```python
from build123d import *

# Parameters (mm, degrees)
SKETCH_1_W           = 30
SKETCH_1_H           = 30
EXTRUDE_1_DEPTH      = 30
SKETCH_34_W          = 20
SKETCH_34_H          = 20
CUT_EXTRUDE_23_DEPTH = 52.961524227
SKETCH_35_W          = 10
SKETCH_35_H          = 10
CUT_EXTRUDE_24_DEPTH = 47.904157598
CUT_EXTRUDE_25_DEPTH = 47.904157598


with BuildPart() as part:
    # 草圖1 → 填料-伸1 (new body)
    with BuildSketch(Plane.XY):
        with Locations((15, 15)):
            Rectangle(SKETCH_1_W, SKETCH_1_H)
    extrude(amount=-EXTRUDE_1_DEPTH)

    # 草圖34 → 除料-伸長23 (cut, through all)
    with BuildSketch(Plane.XY):
        with Locations((20, 20)):
            Rectangle(SKETCH_34_W, SKETCH_34_H)
    extrude(amount=-CUT_EXTRUDE_23_DEPTH, mode=Mode.SUBTRACT)

    # 草圖35 → 除料-伸長24 (cut, through all)
    with BuildSketch(Plane(origin=(10, 0, 0), x_dir=(0, 0, -1), z_dir=(1, 0, 0))):
        with Locations((5, 25)):
            Rectangle(SKETCH_35_W, SKETCH_35_H)
    extrude(amount=-CUT_EXTRUDE_24_DEPTH, mode=Mode.SUBTRACT)

    # 草圖36 → 除料-伸長25 (cut, through all)
    with BuildSketch(Plane(origin=(0, 10, 0), x_dir=(1, 0, 0), z_dir=(0, 1, 0))):
        Polygon((10, 0), (30, 20), (30, 0), align=None)
    extrude(amount=-CUT_EXTRUDE_25_DEPTH, mode=Mode.SUBTRACT)


solid = part.part
```
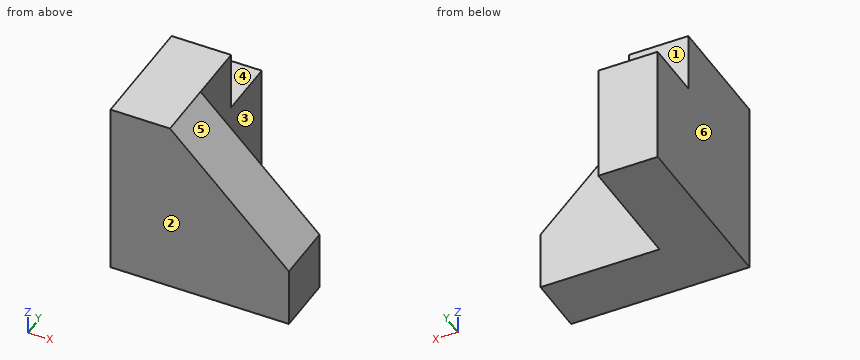
Geometry: final body of the model. Coordinates: model frame, mm. Face numbers are marked on the shaded views. A direction names the side the tool comes from. Give positions to 0.01 mm unless a question says otherwise; leave off trailing zeros. Loops run counter-clockwise (first coordinate to the right, second up) from the corner with the lowest first, then second, coordinate; pieces in that order, holes last. Notation, with made-up numbers: (50.25, 12) - (59.25, 12) arc R8 ccw to (59.25, 27) - close; hole circle Ø11 at (-7.5, 78). An arc over 180 degrees is marked (long way). Answer as CSV lines item,"result". Start each with the question number.
(1) Section query D-D (x = 15.5). Output: boundary loops of the cut face in (y, z).
(2) Mould query, pull axis X, two halves, no side actions, for the marked faces 4, 5 and 6. Classes: +X half, -X half, draft (parallel to the pull), parting line (faces both ways), or undercut.
(3) Ray query, line 1 along X through (y, z) = (14, -9.25); line 2 along Z through (x, y) = (6.5, 25). Return the intervals inside material, ascending. Write a range as [from, to].
(4) Section query B-B (z = -19). Output: boundary loops of the cut face in (x, y).
(5) Section query A-A (x = 3). Output: boundary loops of the cut face in (y, z).
(6) Section query C-C (y = 5.75). Output: boundary loops of the cut face in (x, z).
(7) Pin query (flat end, axial travel): P1, Ø2, axis at y = 9.5, z = -6.5, coming from the +X side; P2, Ø16, axis at x = 18.5, z = -18.5, coming from the +Y side; P3, Ø3, axis at x = 20.5, y = 6, coming from the +Z side. Return the tip coordinate at first contact, or that it passes through.
(8) Reachability of the marked faces 1, 2 and 3 from +Z, -Z, +X, -X, +Y, -Y: full face, straight path, thin tool, end or side. Return the list, or none.
Worked answers:
1,outline,"(0, -30) - (10, -30) - (10, -5.5) - (0, -5.5) - close"
2,face 4,"draft"
2,face 5,"+X half"
2,face 6,"-X half"
3,line 1,"x = [0, 10]"
3,line 2,"z = [-30, -10]"
4,outline,"(0, 0) - (29, 0) - (29, 10) - (10, 10) - (10, 30) - (0, 30) - close"
5,outline,"(0, -30) - (30, -30) - (30, -10) - (20, -10) - (20, 0) - (0, 0) - close"
6,outline,"(0, -30) - (30, -30) - (30, -20) - (10, 0) - (0, 0) - close"
7,P1,"stops at x = 17.5"
7,P2,"stops at y = 10"
7,P3,"stops at z = -9"
8,face 1,"+Z, +X, -X, +Y"
8,face 2,"+Z, -Z, +X, -X, -Y"
8,face 3,"+Z, -Z, +X, +Y"
